Build history of the part. All positions in model axes, mm. Round coordinates to 2 decimals unless told otherwise and drop trailing zeros. Write each loop counter-clockwise with the first axis right and the second up, starting at its lowest first coordinate (ties: lowest second). Pieces come first, ordered by that corner, then holes.
1) Saw through at B-B (x = -32). Write the cut outline in (y, z) (3 decimals), plus the area to 3 significant figures.
2) Flat gauge pin, fed straight in: pin 1 (1.9 mm diameter, centred on x = 93.5, z = -1, fed in from -Y) (3 decimals). Where does the tip first touch, or does it go through?
3) Wall check: probe 1 along Y at (x, z) = (-215.9, 5); probe 2 along Y at (x, z) = (-205, 1.25) (3 decimals); probe 3 along Z at (x, y) = (-105, -3.75) (3 decimals). Give the ranges that are in metal, low to high.
4) Saw through at A-A (x = -161). Write the cut outline in (y, z) (3 decimals), plus the area to 3 significant figures.
from build123d import *

# Parameters (mm, degrees)
F0_W          = 457.2
F0_H          = 25.4
F1_DEPTH      = 6.35
F2_R          = 12.69999
F3_R          = 4.7625
F4_DEPTH      = 12.701
F5_W          = 19.05
F5_H          = 6.35
F6_DEPTH      = 228.601
F6_DEPTH_BACK = 228.601
F7_W          = 304.8
F7_H          = 6.35
F8_DEPTH      = 12.701
F9_R          = 3.17499


# Not quite as in the source:
# - a fillet or chamfer is up to 0.001 mm smaller than in the source, because OpenCascade refuses the exact size


with BuildPart() as f1:
    # F0 (on Top) → F1 (new body, symmetric)
    with BuildSketch(Plane.XY):
        Rectangle(F0_W, F0_H)
    extrude(amount=F1_DEPTH, both=True)

    # F2 (radius 12.7 in the source; OpenCascade refuses exactly that, so slightly less here)
    f2_edges = [f1.edges().sort_by_distance(p)[0] for p in [
        (-228.6, 12.7, 0),
        (-228.6, -12.7, 0),
    ]]
    fillet(f2_edges, radius=F2_R)

    # F3 (on face) → F4 (cut, through all)
    with BuildSketch(Plane(origin=(0, 0, -6.35), x_dir=(1, 0, 0), z_dir=(0, 0, -1))):
        with Locations((-215.9, 0)):
            Circle(F3_R)
    extrude(amount=-F4_DEPTH, mode=Mode.SUBTRACT)

    # F5 (on Right) → F6 (cut, two sides)
    with BuildSketch(Plane.YZ) as f6_sk:
        Rectangle(F5_W, F5_H)
    extrude(amount=-F6_DEPTH, mode=Mode.SUBTRACT)
    extrude(f6_sk.sketch, amount=F6_DEPTH_BACK, mode=Mode.SUBTRACT)

    # F7 (on Front) → F8 (cut, through all)
    with BuildSketch(Plane.XZ):
        with Locations((50.8, 0)):
            Rectangle(F7_W, F7_H)
    extrude(amount=F8_DEPTH, mode=Mode.SUBTRACT)

    # F9 (radius 3.175 in the source; OpenCascade refuses exactly that, so slightly less here)
    f9_edges = [f1.edges().sort_by_distance(p)[0] for p in [
        (-101.6, -11.1125, 3.175),
        (203.2, -11.1125, -3.175),
        (203.2, -11.1125, 3.175),
        (-101.6, -11.1125, -3.175),
    ]]
    fillet(f9_edges, radius=F9_R)


solid = f1.part
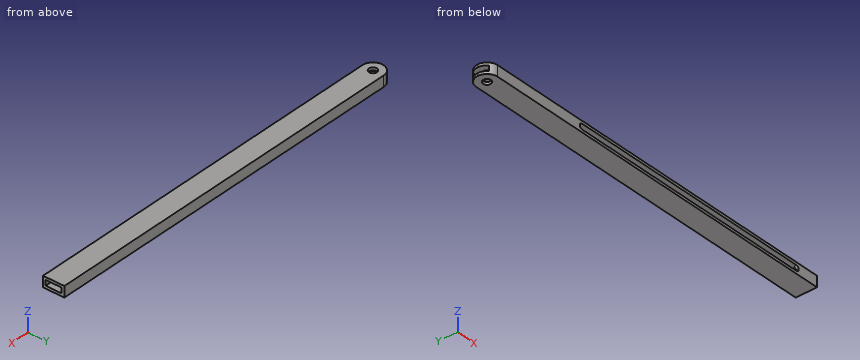
Evaluation:
1. outline: (-12.7, -6.35) - (12.7, -6.35) - (12.7, 6.35) - (-12.7, 6.35) - (-12.7, 3.175) - (9.525, 3.175) - (9.525, -3.175) - (-12.7, -3.175) - close
1. area: 181 mm2
2. pin 1: stops at y = 9.525
3. probe 1: y = -12.7 to -4.76, 4.76 to 12.7
3. probe 2: y = -12.7 to -9.525, 9.525 to 12.7
3. probe 3: z = -6.35 to -3.175, 3.175 to 6.35
4. outline: (-12.7, -6.35) - (12.7, -6.35) - (12.7, 6.35) - (-12.7, 6.35) - close; hole (-9.525, -3.175) - (9.525, -3.175) - (9.525, 3.175) - (-9.525, 3.175) - close
4. area: 202 mm2
